Geometry check sheet. Reference: the model listing, model coordinates, mm. Coordinates: 2 decimals unless noted, no trailing zeros. Loops run counter-clockwise (first coordinate to the right, second up) from the corner with the lowest first, then second, coordinate; pieces in that order, holes last. Notation, with made-up numbers: (31.25, 63.25) -> (81.25, 63.25) arc R27 ccw to (81.25, 96.25) -> close; hole circle Ø9 at (62, 32). An arc over 180 degrees is marked (long way). Answer as a JSON object with one key per item and string values.
Autodesk Fusion 360 part; units mm, degrees
sketch "Sketch1" plane through (0, 0, 0) normal (0, 0, 1) x (1, 0, 0)
  line L0 (0, 0) -> (101.6, 0)
  line L1 (101.6, 0) -> (101.6, 73.66)
  line L2 (101.6, 73.66) -> (0, 73.66)
  line L3 (0, 73.66) -> (0, 0)
  dimension "d1" = 101.6
  dimension "d2" = 73.66
extrude "Extrude1" add sketch "Sketch1" along normal blind 1.5
sketch "Sketch2" plane through (0, 0, 1.5) normal (0, 0, 1) x (-1, 0, 0)
  line L0 (0, -73.66) -> (0, 0)
  line L1 (0, 0) -> (-101.6, 0)
  line L2 (-101.6, 0) -> (-101.6, -73.66)
  line L3 (-101.6, -73.66) -> (0, -73.66)
  line L4 (-10, -35) -> (-25, -35)
  line L5 (-10, -30) -> (-25, -30)
  line L6 (-35, -35) -> (-50, -35)
  line L7 (-35, -30) -> (-50, -30)
  line L8 (-60, -35) -> (-75, -35)
  line L9 (-85, -35) -> (-95, -35)
  line L10 (-60, -30) -> (-75, -30)
  line L11 (-85, -30) -> (-95, -30)
  line L12 (-25, -55) -> (-10, -55)
  line L13 (-50, -55) -> (-35, -55)
  line L14 (-95, -55) -> (-85, -55)
  line L15 (-75, -55) -> (-60, -55)
  line L16 (-85, -10) -> (-95, -10)
  line L17 (-60, -10) -> (-75, -10)
  line L18 (-10, -10) -> (-25, -10)
  line L19 (-35, -10) -> (-50, -10)
  line L20 (-10, -20) -> (-95, -20)
  line L21 (-10, -15) -> (-95, -15)
  line L22 (-25, -30) -> (-25, -20)
  line L23 (-25, -15) -> (-25, -10)
  line L24 (-10, -10) -> (-10, -15)
  line L25 (-10, -20) -> (-10, -30)
  line L26 (-35, -30) -> (-35, -20)
  line L27 (-35, -15) -> (-35, -10)
  line L28 (-50, -30) -> (-50, -20)
  line L29 (-50, -15) -> (-50, -10)
  line L30 (-60, -30) -> (-60, -20)
  line L31 (-60, -15) -> (-60, -10)
  line L32 (-75, -30) -> (-75, -20)
  line L33 (-75, -15) -> (-75, -10)
  line L34 (-85, -30) -> (-85, -20)
  line L35 (-85, -15) -> (-85, -10)
  line L36 (-95, -30) -> (-95, -20)
  line L37 (-95, -15) -> (-95, -10)
  line L38 (-10, -35) -> (-10, -42.8011)
  line L39 (-10, -47.4728) -> (-10, -55)
  line L40 (-25, -55) -> (-25, -47.4728)
  line L41 (-25, -42.8011) -> (-25, -35)
  line L42 (-35, -55) -> (-35, -47.4728)
  line L43 (-35, -42.8011) -> (-35, -35)
  line L44 (-10, -42.8011) -> (-25, -42.8011)
  line L45 (-10, -47.4728) -> (-25, -47.4728)
  line L46 (-35, -47.4728) -> (-50, -47.4728)
  line L47 (-35, -42.8011) -> (-50, -42.8011)
  line L48 (-50, -55) -> (-50, -47.4728)
  line L49 (-50, -42.8011) -> (-50, -35)
  line L50 (-60, -55) -> (-60, -47.4728)
  line L51 (-60, -42.8011) -> (-60, -35)
  line L52 (-60, -47.4728) -> (-75, -47.4728)
  line L53 (-85, -47.4728) -> (-95, -47.4728)
  line L54 (-75, -55) -> (-75, -47.4728)
  line L55 (-75, -42.8011) -> (-75, -35)
  line L56 (-60, -42.8011) -> (-75, -42.8011)
  line L57 (-85, -42.8011) -> (-95, -42.8011)
  line L58 (-85, -55) -> (-85, -47.4728)
  line L59 (-85, -42.8011) -> (-85, -35)
  line L60 (-95, -55) -> (-95, -47.4728)
  line L61 (-95, -42.8011) -> (-95, -35)
extrude "Extrude2" cut sketch "Sketch2" against normal blind 5 contours L4 L38 L41 L44 | L11 L20 L34 L36 | L10 L20 L30 L32 | L7 L20 L26 L28 | L5 L20 L22 L25 | L6 L43 L47 L49 | L8 L51 L55 L56 | L9 L57 L59 L61 | L12 L39 L40 L45 | L13 L42 L46 L48 | L14 L53 L58 L60 | L15 L50 L52 L54 | L16 L21 L35 L37 | L18 L21 L23 L24 | L19 L21 L27 L29 | L17 L21 L31 L33
1. Section check B-B, the plane x = 91. Record the boundary of the cut face in (y, z).
Evaluation:
{"outline": "(0, 0) -> (10, 0) -> (10, 1.5) -> (0, 1.5) -> close; (15, 0) -> (20, 0) -> (20, 1.5) -> (15, 1.5) -> close; (30, 0) -> (35, 0) -> (35, 1.5) -> (30, 1.5) -> close; (42.8, 0) -> (47.47, 0) -> (47.47, 1.5) -> (42.8, 1.5) -> close; (55, 0) -> (73.66, 0) -> (73.66, 1.5) -> (55, 1.5) -> close"}
2. Section check C-C, the plane z = 1.1. State how many separate pieces and enclosed holes the cut face has, then the cut area to 3 significant figures.
Evaluation:
{"separate pieces": "1", "enclosed holes": "16", "area": "5,820 mm^2"}
3. Thickness scan on probe 1 along Y at (x, z) = (24, 0.45); probe 2 along X at (y, z) = (25.5, 1.3). Record the ranges inside material, lowest first. Write a range as from..to.
Evaluation:
{"probe 1": "y = 0..10, 15..20, 30..35, 42.8..47.47, 55..73.66", "probe 2": "x = 0..10, 25..35, 50..60, 75..85, 95..101.6"}
4. Section check A-A, the plane y = 28.5. Record the boundary of the cut face in (x, z).
Evaluation:
{"outline": "(0, 0) -> (10, 0) -> (10, 1.5) -> (0, 1.5) -> close; (25, 0) -> (35, 0) -> (35, 1.5) -> (25, 1.5) -> close; (50, 0) -> (60, 0) -> (60, 1.5) -> (50, 1.5) -> close; (75, 0) -> (85, 0) -> (85, 1.5) -> (75, 1.5) -> close; (95, 0) -> (101.6, 0) -> (101.6, 1.5) -> (95, 1.5) -> close"}
